Could you check a few things on this model? Use its own coordinates, in mm. Face numbers are marked on the shaded views. A direction names the side the tool comes from. Give positions to 0.01 mm unless a question says otherwise; leave off trailing zeros. Order: outer loops, then holes, each group sorted by start corner. A loop starts at its lowest first (then second) coordinate and runs counter-clockwise, first axis right, second up. Notation, with made-up numbers: M 36,38.25 L 84,38.25 A23 cw 84,47.25 Z; hole C 89.5,40.5 d11. An arc over 180 degrees is marked long. Use a Markdown table: item, result. Add a question column.
Item 1: Suppose I cut it at C-C on y = -6. Write out the boundary of the cut face in (x, z) (3 decimals), plus the area to 3 significant figures.
Item 2: Suppose I cut it at A-A on z = 0. Write out the boundary of the cut face in (x, y) (3 decimals), plus the area to 3 significant figures.
Item 3: I'm going to push flat-ended pins straight in: pin 1 Ø2.5 at (x, z) = (27.26, 33.61) entering from -Y; pin 2 Ø2 at (y, z) = (-29, -8.5) entering from +X; pin 3 Ø9 at (y, z) = (-65, 0.5) entering from -X; pin 4 Ø9 at (x, y) = (-0.5, -30.5) entering from -Z. Where does each tip first touch, or does it pass through?
Item 4: Suppose I cut it at D-D on z = 8. Write out the boundary of the cut face in (x, y) (3 decimals).
Item 5: If we mould it in two halves opening along X, with no side actions, what happens to the marked faces 5, 6 and 7? For each: released by +X, released by -X, zero draft, split by the parting line, or undercut.
Item 6: For the marked faces 1, 2, 3 and 4, which set-ups out of +Z, -Z, +X, -X, +Y, -Y let a thin tool reach every point of the face, with its end or its side?
Item 7: Suppose I cut it at B-B on y = -76.2. Write out the boundary of the cut face in (x, z) (3 decimals), plus the area to 3 significant figures.
Item 8: If I drill on L1, parallel to Z at x = -10, y = -16; L2, parallel to Y at x = -27.5, z = 21 (3 decimals), over which ranges is the centre line in solid material (lowest first)? Write a range as from..to.
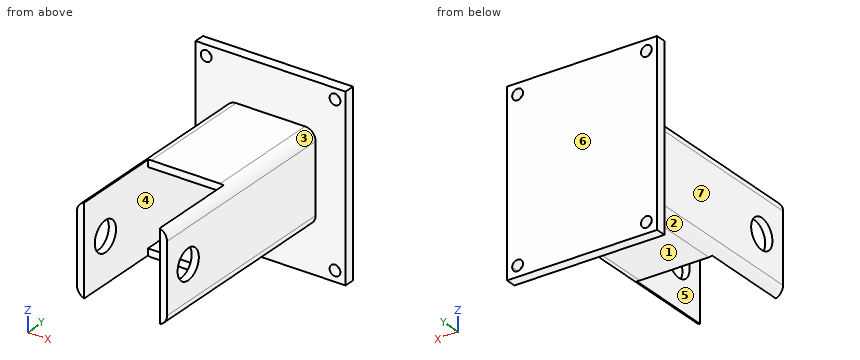
from build123d import *

# Parameters (mm, degrees)
F0_W      = 32.004
F0_H      = 32.004
F1_DEPTH  = 88.9
F2_R      = 6.35
F3_DEPTH  = 24.384
F5_W      = 32.004
F5_H      = 50.8
F6_DEPTH  = 38.1
F7_W      = 63.5
F7_H      = 76.2
F8_DEPTH  = 4.445
F9_R      = 2.286
F10_DEPTH = 25.4


with BuildPart() as f1:
    # F0 (on Front) → F1 (new body)
    with BuildSketch(Plane.XZ):
        with BuildLine():
            ThreePointArc((19.05, 14.605), (17.74809, 17.74809), (14.605, 19.05))
            Line((14.605, 19.05), (-14.605, 19.05))
            ThreePointArc((-14.605, 19.05), (-17.74809, 17.74809), (-19.05, 14.605))
            Line((-19.05, 14.605), (-19.05, -14.605))
            ThreePointArc((-19.05, -14.605), (-17.74809, -17.74809), (-14.605, -19.05))
            Line((-14.605, -19.05), (14.605, -19.05))
            ThreePointArc((14.605, -19.05), (17.74809, -17.74809), (19.05, -14.605))
            Line((19.05, -14.605), (19.05, 14.605))
        make_face()
        Rectangle(F0_W, F0_H, mode=Mode.SUBTRACT)
    extrude(amount=F1_DEPTH)

    # F2 (on Right) → F3 (cut, symmetric)
    with BuildSketch(Plane.YZ):
        with Locations((-76.2, 0)):
            Circle(F2_R)
    extrude(amount=F3_DEPTH, both=True, mode=Mode.SUBTRACT)

    # F5 (on offset) → F6 (cut)
    with BuildSketch(Plane.XZ.offset(88.9)):
        Rectangle(F5_W, F5_H)
    extrude(amount=-F6_DEPTH, mode=Mode.SUBTRACT)

    # F7 (on Front) → F8 (join)
    with BuildSketch(Plane.XZ):
        Rectangle(F7_W, F7_H)
    extrude(amount=-F8_DEPTH)

    # F9 (on face) → F10 (cut)
    with BuildSketch(Plane.XZ):
        with Locations((27.259872, 33.609872)):
            Circle(F9_R)
        with BuildLine():
            ThreePointArc((28.876318, -35.226318), (29.371861, -34.484686), (29.545872, -33.609872))
            ThreePointArc((29.545872, -33.609872), (25.147883, -32.735058), (28.876318, -35.226318))
        make_face()
        with Locations((-27.259872, -33.609872)):
            Circle(F9_R)
        with Locations((-27.259872, 33.609872)):
            Circle(F9_R)
    extrude(amount=-F10_DEPTH, mode=Mode.SUBTRACT)


solid = f1.part
Findings below:
| question | item | result |
|---|---|---|
| 1 | outline | M -19.05,-14.605 A4.445 ccw -14.605,-19.05 L 14.605,-19.05 A4.445 ccw 19.05,-14.605 L 19.05,14.605 A4.445 ccw 14.605,19.05 L -14.605,19.05 A4.445 ccw -19.05,14.605 Z; hole M -16.002,-16.002 L 16.002,-16.002 L 16.002,16.002 L -16.002,16.002 Z |
| 1 | area | 410 mm^2 |
| 2 | outline | M -31.75,0 L -19.05,0 L -19.05,-69.85 L -16.002,-69.85 L -16.002,0 L 16.002,0 L 16.002,-69.85 L 19.05,-69.85 L 19.05,0 L 31.75,0 L 31.75,4.445 L -31.75,4.445 Z; M -19.05,-88.9 L -16.002,-88.9 L -16.002,-82.55 L -19.05,-82.55 Z; M 16.002,-88.9 L 19.05,-88.9 L 19.05,-82.55 L 16.002,-82.55 Z |
| 2 | area | 747 mm^2 |
| 3 | pin 1 | passes through |
| 3 | pin 2 | stops at x = 19.05 |
| 3 | pin 3 | stops at x = -19.05 |
| 3 | pin 4 | stops at z = -19.05 |
| 4 | outline | M -31.75,0 L -19.05,0 L -19.05,-88.9 L -16.002,-88.9 L -16.002,0 L 16.002,0 L 16.002,-88.9 L 19.05,-88.9 L 19.05,0 L 31.75,0 L 31.75,4.445 L -31.75,4.445 Z |
| 5 | face 5 | undercut |
| 5 | face 6 | zero draft |
| 5 | face 7 | released by -X |
| 6 | face 1 | -Z, +X, -X, -Y |
| 6 | face 2 | -Z, -X, -Y |
| 6 | face 3 | +Z, +X, -Y |
| 6 | face 4 | -Y |
| 7 | outline | M -19.05,-14.605 A4.445 ccw -16.002,-18.825 L -16.002,-6.35 L -19.05,-6.35 Z; M -19.05,6.35 L -16.002,6.35 L -16.002,18.825 A4.445 ccw -19.05,14.605 Z; M 16.002,-18.825 A4.445 ccw 19.05,-14.605 L 19.05,-6.35 L 16.002,-6.35 Z; M 16.002,6.35 L 19.05,6.35 L 19.05,14.605 A4.445 ccw 16.002,18.825 Z |
| 7 | area | 138 mm^2 |
| 8 | L1 | z = -19.05..-16, 16..19.05 |
| 8 | L2 | y = 0..4.445 |
